from build123d import *

# Parameters (mm, degrees)
F0_R     = 7.9375
F0_R_2   = 3.556
F1_DEPTH = 12.7
F2_R     = 1.27
F3_DEPTH = 7.9385
F5_R     = 3.556
F6_DEPTH = 5.334


with BuildPart() as f1:
    # F0 (on Top) → F1 (new body)
    with BuildSketch(Plane.XY):
        Circle(F0_R)
        Circle(F0_R_2, mode=Mode.SUBTRACT)
    extrude(amount=F1_DEPTH)

    # F2 (on Front) → F3 (cut, through all)
    with BuildSketch(Plane.XZ):
        with Locations((0, 6.35)):
            Circle(F2_R)
    extrude(amount=-F3_DEPTH, mode=Mode.SUBTRACT)

    # F5 (on offset) → F6 (cut)
    with BuildSketch(Plane.XZ.offset(-11.1125)):
        with Locations((0, 6.35)):
            Circle(F5_R)
    extrude(amount=F6_DEPTH, mode=Mode.SUBTRACT)


solid = f1.part
Read the model definition and answer for the solid it produces. Units are mm, in the model's axes. A direction names the side the tool comes from. Round coordinates to 2 decimals unless told otherwise and drop trailing zeros. Write each loop counter-clockwise with the first axis right and the second up, starting at its lowest first coordinate (ties: lowest second). Pieces come first, ordered by that corner, then holes. Notation, with made-up numbers: M -33,34.5 L 13,34.5 A21 cw 13,61.5 Z; hole C -32,-19 d3. An arc over 180 degrees is marked long. Use a Markdown table: item, result.
1) A tool of negligible diameter and unlimited length cuts with its end or side. For faces 5 (the cylindrical face through (-0.77, -3.47, 6.26)), 6 (the flat face through (0, 5.779, 4.8)), from which of +Z, -Z, +X, -X, +Y, -Y can it reach the whole face along a straight path? Write none if from no direction.
Answers follow:
| item | result |
|---|---|
| face 5 | +Z, -Z |
| face 6 | +Y |
2) Flat-ended cylindrical pins translate along their axes: pin 1 (2 mm diameter, centred on y = 4.5, z = 8.5, fed in from -X); pin 2 (6 mm diameter, centred on y = -1.5, z = 5, fed in from +X); pin 3 (5 mm diameter, centred on y = -4, z = 3, fed in from +X); pin 4 (1 mm diameter, centred on x = -6, z = 7, fed in from +Y). Find the tip coordinate at first contact, or state that the pin passes through.
Answers follow:
| item | result |
|---|---|
| pin 1 | stops at x = -7.12 |
| pin 2 | stops at x = 7.94 |
| pin 3 | stops at x = 7.79 |
| pin 4 | stops at y = 5.72 |
3) The part is cut by section D-D (y = 6.5). Write down the section's boundary in (x, z).
Answers follow:
| item | result |
|---|---|
| outline | M -4.56,0 L 4.56,0 L 4.56,12.7 L -4.56,12.7 Z; hole C 0,6.35 d7.11 |
4) The part is cut by section A-A (x = 0). Write down the section's boundary in (y, z).
Answers follow:
| item | result |
|---|---|
| outline | M -7.94,0 L -3.56,0 L -3.56,12.7 L -7.94,12.7 Z; M 3.56,0 L 7.94,0 L 7.94,2.79 L 5.78,2.79 L 5.78,5.08 L 3.56,5.08 Z; M 3.56,7.62 L 5.78,7.62 L 5.78,9.91 L 7.94,9.91 L 7.94,12.7 L 3.56,12.7 Z |
5) The part is cut by section B-B (y = 0). Write down the section's boundary in (x, z), plus the area to 3 significant figures.
Answers follow:
| item | result |
|---|---|
| outline | M -7.94,0 L -3.56,0 L -3.56,12.7 L -7.94,12.7 Z; M 3.56,0 L 7.94,0 L 7.94,12.7 L 3.56,12.7 Z |
| area | 111 mm2 |
6) The part is cut by section C-C (z = 11). Write down the section's boundary in (x, y) (1 decimal).
Answers follow:
| item | result |
|---|---|
| outline | C 0,0 d15.9; hole C 0,0 d7.1 |
7) For a pull along Z with two mould halves and no side action, classify faces 1 (the flat face through (3.4, -1.7, 12.7)), 2 (the flat face through (3.4, -1.7, 0)), 3 (the cylindrical face through (-1.27, 4.53, 6.41)), 4 (the cylindrical face through (3.285, 6.636, 4.988)) as pulls with the +Z half, pulls with the -Z half, needs draft (parallel to the pull), parting line crosses it, or undercut.
Answers follow:
| item | result |
|---|---|
| face 1 | pulls with the +Z half |
| face 2 | pulls with the -Z half |
| face 3 | undercut |
| face 4 | undercut |
8) Straight lines are drawn through the part: line 1 along Z through (x, y) = (0, 4.05); line 2 along Y through (x, z) = (0, 6); line 3 along X through (y, z) = (2.5, 9.75). For each, find the intervals that lie inside material, in ascending order. Write a range as [from, to].
Answers follow:
| item | result |
|---|---|
| line 1 | z = [0, 5.08], [7.62, 12.7] |
| line 2 | y = [-7.94, -3.56] |
| line 3 | x = [-7.53, -2.53], [2.53, 7.53] |
